Model file for the job. Use its own axes, mm. Round coordinates to 2 decimals unless told otherwise and drop trailing zeros. Loops run counter-clockwise (first coordinate to the right, second up) from the corner with the lowest first, then second, coordinate; pieces in that order, holes last. Notation, with made-up numbers: M 86,76.25 L 109,76.25 A27 ccw 109,115.25 Z; hole C -19.5,66.5 d7. An arc over 180 degrees is marked long. Use a Markdown table: item, result. Add a question column.
Item 1: Saw through at B-B on z = 4.5. Give the number of separate pieces and of enclosed holes in the cut face, then the cut area to 3 significant figures.
Item 2: Wall check: L1, parallel to Y at x = 0, z = 3.25; L2, parallel to Y at x = -3.5, z = 5.75; L3, parallel to X at y = -58.5, z = 3.5. Give the ranges that are in metal, low to high. Write a range as from..to.
Item 3: Saw through at A-A on x = 0. Write the cut outline in (y, z), then the cut area to 3 significant figures.
Item 4: Two-plate mould, pull along X, no slides. Class faces 1 (the cylindrical face through (0.1, 73.247, 3.131)), 2 (the flat face through (0, 20, 0)), 3 (the cylindrical face through (-2.21, 50.77, 3.13)): +X half, -X half, draft (parallel to the pull), parting line (faces both ways), or undercut.
Item 5: Pin check, flat tips, straight feed: P1, Ø2, axis at x = -2.5, z = 4, coming from the -Y side; P2, Ø3, axis at x = -4, z = 5.5, coming from the -Y side; P3, Ø3, axis at y = 23, z = 4.5, coming from the +X side. Stop position of each tip, or through.
```python
from build123d import *

# Parameters (mm, degrees)
F0_R     = 4.8813139191
F0_R_2   = 10.1764917569
F1_DEPTH = 6.35


with BuildPart() as f1:
    # F0 (on Top) → F1 (new body)
    with BuildSketch(Plane.XY):
        with BuildLine():
            add(Edge.make_bspline(
                [(-12.5280236165, 61.3621314645), (-7.3308367109, 16.0433941021), (-2.1616382879, -29.2743790858), (-6.2805634765, -59.8213464213)],
                knots=[0, 0, 0, 0, 0.612325914, 0.612325914, 0.612325914, 0.612325914], degree=3))
            ThreePointArc((-6.2805634765, -59.8213464213), (0.0609906573, -65.418488491), (6.2933783491, -59.7000401142))
            add(Edge.make_bspline(
                [(12.5064774979, 61.6896377928), (6.6850781441, 15.9770144044), (0.8078775975, -29.741100788), (6.2933783491, -59.7000401142)],
                knots=[0, 0, 0, 0, 0.6137866635, 0.6137866635, 0.6137866635, 0.6137866635], degree=3))
            ThreePointArc((12.5064774979, 61.6896377928), (-0.1641071527, 73.2467040487), (-12.5280236165, 61.3621314645))
        make_face()
        with Locations((0, -59.0965338051)):
            Circle(F0_R, mode=Mode.SUBTRACT)
        with Locations((0, 60.7023946941)):
            Circle(F0_R_2, mode=Mode.SUBTRACT)
    extrude(amount=F1_DEPTH)


solid = f1.part
```
Entries:
| question | item | result |
|---|---|---|
| 1 | separate pieces | 1 |
| 1 | enclosed holes | 2 |
| 1 | area | 1,580 mm2 |
| 2 | L1 | -65.42..-63.98, -54.22..50.53, 70.88..73.25 |
| 2 | L2 | -64.36..-62.5, -55.69..51.15, 70.26..72.75 |
| 2 | L3 | -6.11..-4.84, 4.84..6.08 |
| 3 | outline | M -65.42,0 L -63.98,0 L -63.98,6.35 L -65.42,6.35 Z; M -54.22,0 L 50.53,0 L 50.53,6.35 L -54.22,6.35 Z; M 70.88,0 L 73.25,0 L 73.25,6.35 L 70.88,6.35 Z |
| 3 | area | 689 mm2 |
| 4 | face 1 | parting line |
| 4 | face 2 | draft |
| 4 | face 3 | undercut |
| 5 | P1 | y = -65.24 |
| 5 | P2 | y = -64.9 |
| 5 | P3 | x = 7.95 |
